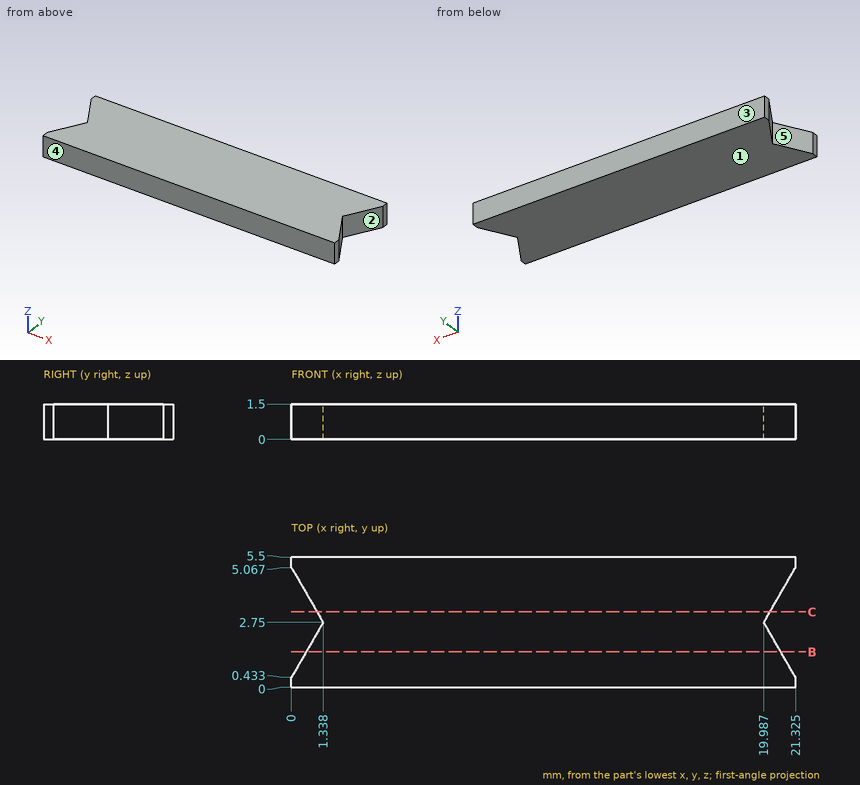
Can you work these out from the drawing? Everything is in mm from the part's minimum corner. A direction names the side the tool comes from. Coordinates: 2 decimals unless noted, no trailing zeros. Write each loop counter-clockwise with the first axis right and the second up, starting at its lowest first coordinate (ties: lowest second). Pieces come first, ordered by that corner, then holes. Notation, with made-up numbers: (79.25, 11.25) - (88.25, 11.25) arc R26 cw to (88.25, 45.25) - close; hole circle Ø2 at (60.25, -16). An arc over 180 degrees is marked (long way). One line per item, written item: value.
1) Suppose I cut it at B-B on y = 1.5. Write out the boundary of the cut face in (x, z).
Model answer:
outline: (0.62, 0) - (20.71, 0) - (20.71, 1.5) - (0.62, 1.5) - close
2) I'm going to push a flat-ended pin straight in: P1, Ø2, axis at x = 14.5, y = 3, coming from the -Z side. Where does the tip first touch, or does it pass through?
Model answer:
P1: stops at z = 0
3) Suppose I cut it at C-C on y = 3.2. Write out the boundary of the cut face in (x, z).
Model answer:
outline: (1.08, 0) - (20.25, 0) - (20.25, 1.5) - (1.08, 1.5) - close
4) We'd pull the mould along Y, two halves only. Please class the marked faces 3, 4 and 5: pulls with the +Y half, pulls with the -Y half, needs draft (parallel to the pull), parting line crosses it, or undercut.
Model answer:
face 3: pulls with the +Y half
face 4: pulls with the -Y half
face 5: undercut
5) On a 3-axis mill with a long thin cutter (end or side, diameter ignored), from which of +Z, -Z, +X, -X, +Y, -Y can I reach the whole of each face in a straight line? I mean the marked faces 1 and 2. Say none if no direction works.
Model answer:
face 1: -Z, +X, -X, +Y, -Y
face 2: +Z, -Z, +X
6) I need wall thicknesses on line 1 along X through (y, z) = (1.9, 0.4); line 2 along X through (y, z) = (2.7, 1) (1 decimal). Which ranges of each line are inside material? Lowest first, please.
Model answer:
line 1: x = 0.85 to 20.48
line 2: x = 1.3 to 20
